Here's the drawing with two shaded views (mm, measured from the low corner). I have some questions. A direction names the side the tool comes from. Round coordinates to 2 decimals unless told otherwise and drop trailing zeros. Loops run counter-clockwise (first coordinate to the right, second up) from the corner with the lowest first, then second, coordinate; pieces in that order, holes last.
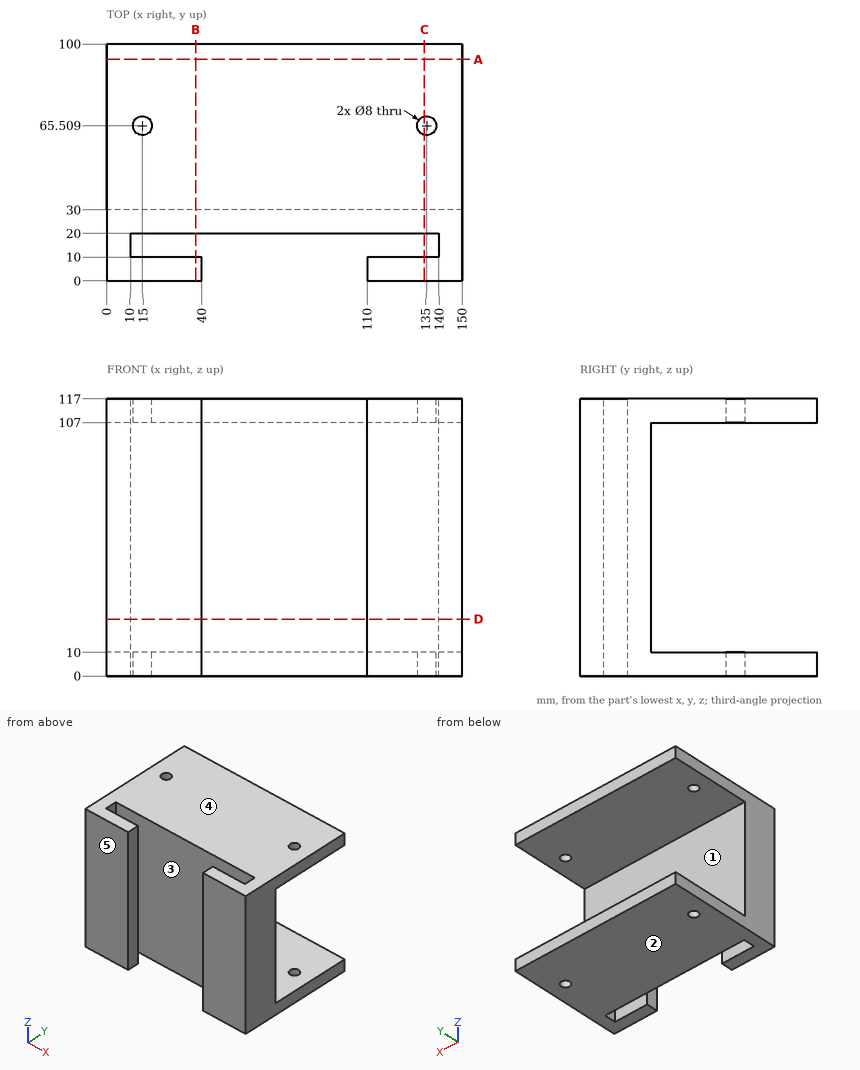
(1) If we section it at D-D, the plane z = 24: List the corners of the cut face in (x, y) for me.
Worked answers:
outline: (0, 0) - (40, 0) - (40, 10) - (10, 10) - (10, 20) - (140, 20) - (140, 10) - (110, 10) - (110, 0) - (150, 0) - (150, 30) - (0, 30) - close
(2) If we mould it in two halves opening along Y, with no side actions, what happens to the marked faces 3, 4 and 5? For each: released by +Y, released by -Y, zero draft, split by the parting line, or undercut.
Worked answers:
face 3: undercut
face 4: zero draft
face 5: released by -Y
(3) If we section it at C-C, the plane x = 134: List the corners of the cut face in (y, z) for me.
Worked answers:
outline: (0, 0) - (10, 0) - (10, 117) - (0, 117) - close; (20, 0) - (61.64, 0) - (61.64, 10) - (30, 10) - (30, 107) - (61.64, 107) - (61.64, 117) - (20, 117) - close; (69.38, 0) - (100, 0) - (100, 10) - (69.38, 10) - close; (69.38, 107) - (100, 107) - (100, 117) - (69.38, 117) - close
(4) If we section it at B-B, the plane x = 37.5: List the corners of the cut face in (y, z) for me.
Worked answers:
outline: (0, 0) - (10, 0) - (10, 117) - (0, 117) - close; (20, 0) - (100, 0) - (100, 10) - (30, 10) - (30, 107) - (100, 107) - (100, 117) - (20, 117) - close
(5) If I drill on line 1 (Y direction, x = 135, z = 6.75); line 2 (Z direction, x = 76, y = 53); line 3 (Y direction, x = 122, z = 64), over which ranges is the centre line in solid material (lowest first)?
Worked answers:
line 1: y = 0 to 10, 20 to 61.51, 69.51 to 100
line 2: z = 0 to 10, 107 to 117
line 3: y = 0 to 10, 20 to 30
(6) If we section it at A-A, the plane y = 93.5: List the corners of the cut face in (x, z) for me.
Worked answers:
outline: (0, 0) - (150, 0) - (150, 10) - (0, 10) - close; (0, 107) - (150, 107) - (150, 117) - (0, 117) - close
(7) For the marked faces 1 and 2, which set-ups out of +Z, -Z, +X, -X, +Y, -Y let a thin tool reach every point of the face, with its end or its side?
Worked answers:
face 1: +X, -X, +Y
face 2: -Z, +X, -X, +Y, -Y
(8) Will these pins go through, and if not, where does the flat tip stop? P1, Ø15, axis at x = 121, z = 34.5, coming from the +Y side; P2, Ø1, axis at x = 92.5, z = 68, coming from the -Y side; P3, Ø5, axis at x = 135, y = 65.51, coming from the -Z side.
Worked answers:
P1: stops at y = 30
P2: stops at y = 20
P3: passes through
